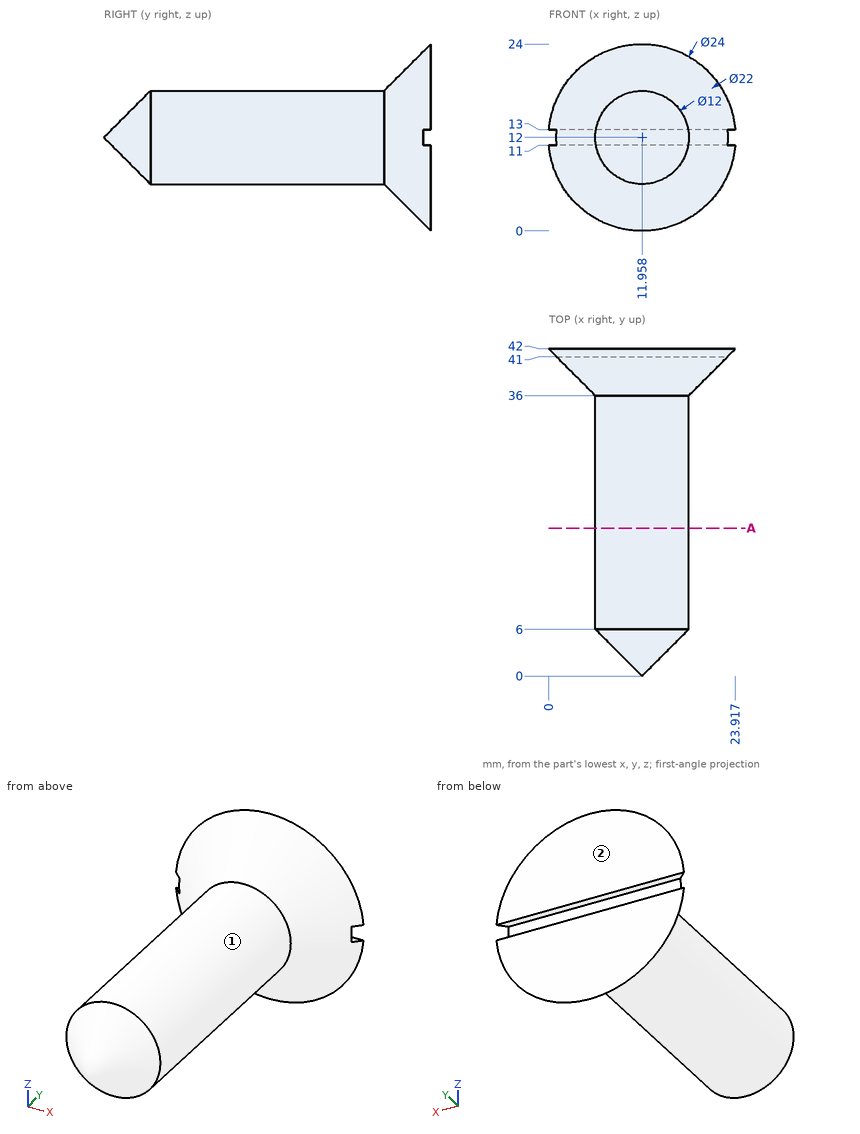
Input: dimensioned drawing with shaded views. Units: mm. Origin: part minimum x, y, z. A direction names the side the tool comes from. Round coordinates to 2 decimals unless told otherwise and drop trailing zeros. Loops run counter-clockwise (first coordinate to the right, second up) from the corner with the lowest first, then second, coordinate; pieces in that order, holes last.
1) Set-up query: the marked faces 1 and 2. Return all of +Z, -Z, +X, -X, +Y, -Y with unobstructed straight access to the full face (end or side cutting, diameter ignored); none if empty.
Ans:
face 1: -Y
face 2: +Z, -Z, +X, -X, +Y
2) Material intervals for line 1 (Z direction, x = 11.75, y = 13.5); line 2 (Y direction, x = 3.5, z = 11.5) (1 decimal); line 3 (Y direction, x = 17.5, z = 6), sorted ascending.
Ans:
line 1: z = 6 to 18
line 2: y = 38.5 to 41
line 3: y = 38.17 to 42
3) Section query A-A on y = 19. Return the cut outline in (x, z), plus the area to 3 significant figures.
Ans:
outline: circle Ø12 at (11.96, 12)
area: 113 mm2
4) Pin query (flat end, axial travel): pin 1 (10 mm diameter, centred on x = 11, y = 5.5, fed in from -Z); pin 2 (1.6 mm diameter, centred on x = 15.5, z = 12, fed in from +Y); pin 3 (5 mm diameter, centred on y = 22, z = 8.5, fed in from +X) (1 decimal). Return the tip coordinate at first contact, or that it passes through.
Ans:
pin 1: stops at z = 6
pin 2: stops at y = 41
pin 3: stops at x = 17.9
